Source: three-view drawing plus pictorial views. Frame: mm from the lowest corner of the part. A direction names the side the tool comes from. Coordinates: 2 decimals unless noted, no trailing zeros. Write each loop counter-clockwise with the first axis right and the second up, starting at its lowest first coordinate (ties: lowest second). Pieces come first, ordered by that corner, then holes.
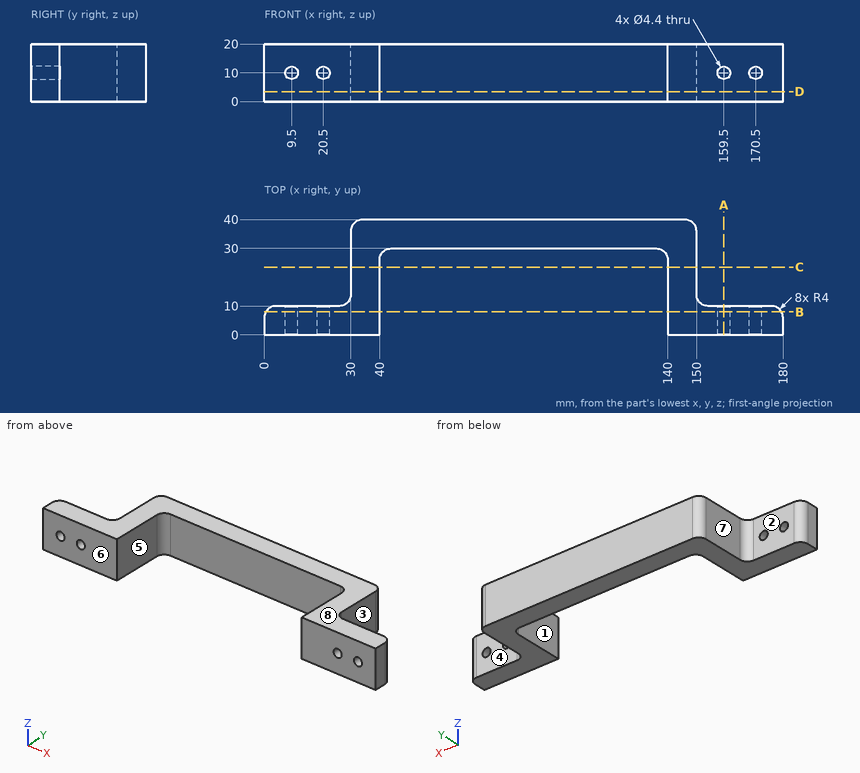
Item 1: Section query C-C, the plane y = 23.5. Return loops of the section in (x, z).
Item 2: Pull-direction query (X, two-part tool) for the marked faces 1, 2 and 3; classes: released by +X, released by -X, zero draft, split by the parting line, or undercut.
Item 3: Material intervals for line 1 (X direction, y = 6.5, z = 10); line 2 (X direction, y = 23.5, z = 17.75); line 3 (X direction, y = 7, z = 10), sorted ascending.
Item 4: Section query D-D, the plane z = 3.5. Return loops of the section in (x, y), then the cut area to 3 significant figures.
Item 5: Access query for the marked faces 4, 5, 6, 7 and 8. Directions: +Z, -Z, +X, -X, +Y, -Y. A direction counts if a zero-diameter tool reaches every point of the face in a straight line with its end or side. Return the directions, or none.
Item 6: Section query B-B, the plane y = 8. Return loops of the section in (x, z), then the cut area to 3 significant figures.
Item 7: Pin query (flat end, axial travel): pin 1 Ø5.5 at (x, z) = (170.5, 10) entering from -Y; pin 2 Ø10 at (y, z) = (20.5, 13) entering from -X; pin 3 Ø5 at (x, z) = (159.5, 10) entering from +Y; pin 4 Ø10 at (x, z) = (113, 14) entering from -Y. Return the tip coordinate at first contact, or that it passes through.
Item 8: Section query A-A, the plane x = 159.5. Return loops of the section in (y, z), then the cut area to 3 significant figures.
The answers:
1. outline: (30, 0) - (40, 0) - (40, 20) - (30, 20) - close; (140, 0) - (150, 0) - (150, 20) - (140, 20) - close
2. face 1: undercut
2. face 2: zero draft
2. face 3: released by +X
3. line 1: x = 0.03 to 7.3, 11.7 to 18.3, 22.7 to 40, 140 to 157.3, 161.7 to 168.3, 172.7 to 179.97
3. line 2: x = 30 to 40, 140 to 150
3. line 3: x = 0.13 to 7.3, 11.7 to 18.3, 22.7 to 40, 140 to 157.3, 161.7 to 168.3, 172.7 to 179.87
4. outline: (0, 0) - (40, 0) - (40, 26) arc R4 cw to (44, 30) - (136, 30) arc R4 cw to (140, 26) - (140, 0) - (180, 0) - (180, 6) arc R4 ccw to (176, 10) - (154, 10) arc R4 cw to (150, 14) - (150, 36) arc R4 ccw to (146, 40) - (34, 40) arc R4 ccw to (30, 36) - (30, 14) arc R4 cw to (26, 10) - (4, 10) arc R4 ccw to (0, 6) - close
4. area: 2,400 mm2
5. face 4: +Z, -Z, +X, +Y
5. face 5: +Z, -Z, -Y
5. face 6: +Z, -Z, +X, -X, -Y
5. face 7: +Z, -Z, -X, +Y
5. face 8: +Z, +X, -X, +Y, -Y
6. outline: (0.54, 0) - (40, 0) - (40, 20) - (0.54, 20) - close; (140, 0) - (179.46, 0) - (179.46, 20) - (140, 20) - close; hole circle Ø4.4 at (9.5, 10); hole circle Ø4.4 at (20.5, 10); hole circle Ø4.4 at (159.5, 10); hole circle Ø4.4 at (170.5, 10)
6. area: 1,520 mm2
7. pin 1: stops at y = 0
7. pin 2: stops at x = 30
7. pin 3: stops at y = 10
7. pin 4: stops at y = 30
8. outline: (0, 0) - (10, 0) - (10, 7.8) - (0, 7.8) - close; (0, 12.2) - (10, 12.2) - (10, 20) - (0, 20) - close
8. area: 156 mm2
